Build history of the part. All positions in model axes, mm. A direction names the side the tool comes from. Round coordinates to 2 decimals unless told otherwise and drop trailing zeros. Write each loop counter-clockwise with the first axis right and the second up, starting at its lowest first coordinate (ties: lowest second). Pieces come first, ordered by that corner, then holes.
from build123d import *

# Parameters (mm, degrees)
SKETCH1_W           = 24.257
SKETCH1_H           = 32.639
BOSS_EXTRUDE1_DEPTH = 2.032
SKETCH2_R           = 0.9525
CUT_EXTRUDE1_DEPTH  = 2.4892
SKETCH3_W           = 22.987
SKETCH3_H           = 23.114
BOSS_EXTRUDE2_DEPTH = 3.556
SKETCH4_R           = 11.4935
BOSS_EXTRUDE3_DEPTH = 11.938
FILLET1_R           = 11.43
SKETCH5_W           = 7.62
SKETCH5_H           = 32.639
BOSS_EXTRUDE4_DEPTH = 8.636
SKETCH6_W           = 3.683
SKETCH6_H           = 7.62
BOSS_EXTRUDE5_DEPTH = 22.86


with BuildPart() as part:
    # Sketch1 → Boss-Extrude1 (new body)
    with BuildSketch(Plane(origin=(0, 0, 0), x_dir=(1, 0, 0), z_dir=(0, 1, 0))):
        Rectangle(SKETCH1_W, SKETCH1_H)
    extrude(amount=BOSS_EXTRUDE1_DEPTH)

    # Sketch2 → Cut-Extrude1 (cut)
    with BuildSketch(Plane(origin=(0, 2.032, 0), x_dir=(1, 0, 0), z_dir=(0, 1, 0))):
        with Locations(Location((0, 14.605, 0), (0, 0, 270))):
            Circle(SKETCH2_R)
        with Locations(Location((0, -14.605, 0), (0, 0, 270))):
            Circle(SKETCH2_R)
    extrude(amount=-CUT_EXTRUDE1_DEPTH, mode=Mode.SUBTRACT)

    # Sketch3 → Boss-Extrude2 (add)
    with BuildSketch(Plane(origin=(0, 2.032, 0), x_dir=(1, 0, 0), z_dir=(0, 1, 0))):
        Rectangle(SKETCH3_W, SKETCH3_H)
    extrude(amount=BOSS_EXTRUDE2_DEPTH)

    # Sketch4 → Boss-Extrude3 (add)
    with BuildSketch(Plane(origin=(0, 5.588, 0), x_dir=(1, 0, 0), z_dir=(0, 1, 0))):
        with Locations(Location((0, 0, 0), (0, 0, 180))):
            Circle(SKETCH4_R)
    extrude(amount=BOSS_EXTRUDE3_DEPTH)

    # Fillet1
    fillet1_edges = [part.edges().sort_by_distance(p)[0] for p in [
        (11.4935, 17.526, 0),
    ]]
    fillet(fillet1_edges, radius=FILLET1_R)

    # Sketch5 → Boss-Extrude4 (add)
    with BuildSketch(Plane.XZ):
        with Locations((8.3185, 0)):
            Rectangle(SKETCH5_W, SKETCH5_H)
    extrude(amount=BOSS_EXTRUDE4_DEPTH)

    # Sketch6 → Boss-Extrude5 (add)
    with BuildSketch(Plane.XZ):
        with Locations((-10.287, -0.28087532)):
            Rectangle(SKETCH6_W, SKETCH6_H)
    extrude(amount=BOSS_EXTRUDE5_DEPTH)


solid = part.part
1) Slice it at B-B (y = -19). Write the cut outline in (x, z).
Results:
outline: (-12.13, -4.09) - (-8.45, -4.09) - (-8.45, 3.53) - (-12.13, 3.53) - close
2) Slice it at A-A (y = -3). Write the cut outline in (x, z).
Results:
outline: (-12.13, -4.09) - (-8.45, -4.09) - (-8.45, 3.53) - (-12.13, 3.53) - close; (4.51, -16.32) - (12.13, -16.32) - (12.13, 16.32) - (4.51, 16.32) - close
3) Wall check: L1, parallel to Y at x = -4.5, z = -2.5; L2, parallel to X at y = -2, z = 15; L3, parallel to X at y = -12, z = -2. Give the ranges that are in metal, low to high.
Results:
L1: y = 0 to 16.33
L2: x = 4.51 to 12.13
L3: x = -12.13 to -8.45
4) Pin check, flat tips, straight feed: pin 1 Ø2 at (x, z) = (0, -14.605) entering from -Y; pin 2 Ø4.5 at (y, z) = (-6, 6) entering from -X; pin 3 Ø4 at (y, z) = (4, 5) entering from +X; pin 4 Ø1.8 at (x, y) = (-10, -10.5) entering from -Z. Stop position of each tip, or through.
Results:
pin 1: stops at y = 0
pin 2: stops at x = 4.51
pin 3: stops at x = 12.13
pin 4: stops at z = -4.09
5) Which spindle directions (+Z, -Z, +X, -X, +Y, -Y) get a long thin tool onto all of the face, cutting with end or side? Do faces 5 (the cylindrical face through (-5.3, 5.8, -10.2)), 6 (the flat face through (11.494, 4, 0)), 7 (the flat face through (-2.6, 5.588, -11.4)), 8 (the flat face through (0, 4, -11.557)). Say none if no direction does.
Results:
face 5: +Y
face 6: +Z, -Z, +X, +Y
face 7: -Z, +Y
face 8: -Z, +X, -X, +Y
6) Mould opens along Z. For faces 1 (the flat face through (4.508, -4, 0)), 2 (the flat face through (0, 4, 11.557)), 3 (the cylindrical face through (0.286, 1.03, 15.514)), 4 (the cylindrical face through (0.3, 1, -13.7)) say: released by +Z, released by -Z, zero draft, split by the parting line, or undercut.
Results:
face 1: zero draft
face 2: released by +Z
face 3: undercut
face 4: undercut
